The listing builds one solid part. Answer for the finished solid, in the listing's coordinates (mm). Face numbers are marked on the shaded views. A direction names the side the tool comes from. Coordinates: 2 decimals unless noted, no trailing zeros. Write each loop counter-clockwise with the first axis right and the second up, starting at its lowest first coordinate (ties: lowest second). Pieces come first, ordered by that corner, then holes.
from build123d import *

# Parameters (mm, degrees)
F0_R     = 7.5
F0_R_2   = 4
F1_DEPTH = 3
F2_R     = 10
F2_R_2   = 7.5
F2_R_3   = 4
F3_DEPTH = 0.5


with BuildPart() as f1:
    # F0 (on Top) → F1 (new body)
    with BuildSketch(Plane.XY):
        Circle(F0_R)
        Circle(F0_R_2, mode=Mode.SUBTRACT)
    extrude(amount=F1_DEPTH)

    # F2 (on face) → F3 (join)
    with BuildSketch(Plane.XY.offset(3)):
        Circle(F2_R)
        Circle(F2_R_2, mode=Mode.SUBTRACT)
        Circle(F2_R_2)
        Circle(F2_R_3, mode=Mode.SUBTRACT)
    extrude(amount=F3_DEPTH)

    # F4: F1 across face


with BuildPart() as f1_1:
    add(f1.part)
    add(f1.part.mirror(Plane(origin=(0, 0, 0), x_dir=(1, 0, 0), z_dir=(0, 0, -1))))


solid = f1_1.part
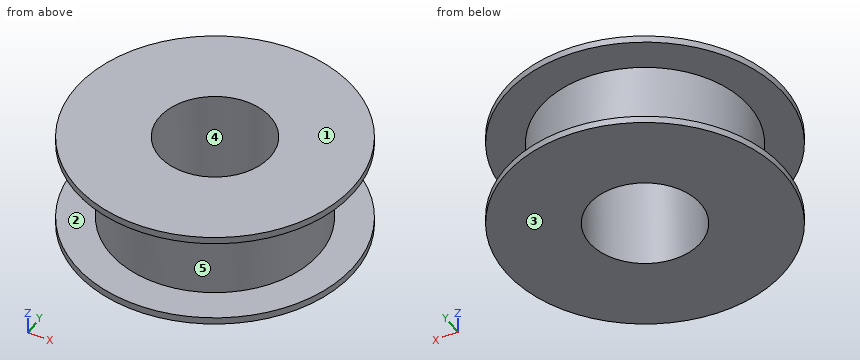
Q1. Determine the mould class of the marked faces 3, 4 and 5 for opening direction Z: released by +Z, released by -Z, zero draft, split by the parting line, or undercut.
Answers below:
face 3: released by -Z
face 4: zero draft
face 5: undercut
Q2. Given pin 1 (4 mm diameter, centred on y = 3.5, z = 0.5, fed in from +X); pin 2 (3 mm diameter, centred on x = -5.5, z = -1, fed in from +Y); pin 3 (7 mm diameter, centred on x = 0, y = 0, fed in from -Z), each flat-ended and moving along its own axis, determine where each tip first touches the part or whether it passes through.
Answers below:
pin 1: stops at x = 7.35
pin 2: stops at y = 6.34
pin 3: passes through
Q3. The part is cut by section A-A, the plane x = 0. Write down the section's boundary in (y, z).
Answers below:
outline: (-10, -3.5) - (-4, -3.5) - (-4, 3.5) - (-10, 3.5) - (-10, 3) - (-7.5, 3) - (-7.5, -3) - (-10, -3) - close; (4, -3.5) - (10, -3.5) - (10, -3) - (7.5, -3) - (7.5, 3) - (10, 3) - (10, 3.5) - (4, 3.5) - close
Q4. The part is cut by section D-D, the plane x = -8. Write down the section's boundary in (y, z), then the cut area to 3 significant figures.
Answers below:
outline: (-6, -3.5) - (6, -3.5) - (6, -3) - (-6, -3) - close; (-6, 3) - (6, 3) - (6, 3.5) - (-6, 3.5) - close
area: 12.0 mm2
Q5. The part is cut by section C-C, the plane z = -2. Write down the section's boundary in (x, y).
Answers below:
outline: circle Ø15 at (0, 0); hole circle Ø8 at (0, 0)
Q6. Which of the six approach directions +Z, -Z, +X, -X, +Y, -Y give full straight-line access (tool end or side, diameter ignored) to the marked faces 1 and 2?
Answers below:
face 1: +Z, +X, -X, +Y, -Y
face 2: none
Q7. Find the intervals of material crossed by probe 1 along Y at (x, z) = (0, 1); probe 2 along Z at (x, y) = (-4.5, -7.5); probe 3 along X at (y, z) = (-1.25, -2.5), in increasing order.
Answers below:
probe 1: y = -7.5 to -4, 4 to 7.5
probe 2: z = -3.5 to -3, 3 to 3.5
probe 3: x = -7.4 to -3.8, 3.8 to 7.4
